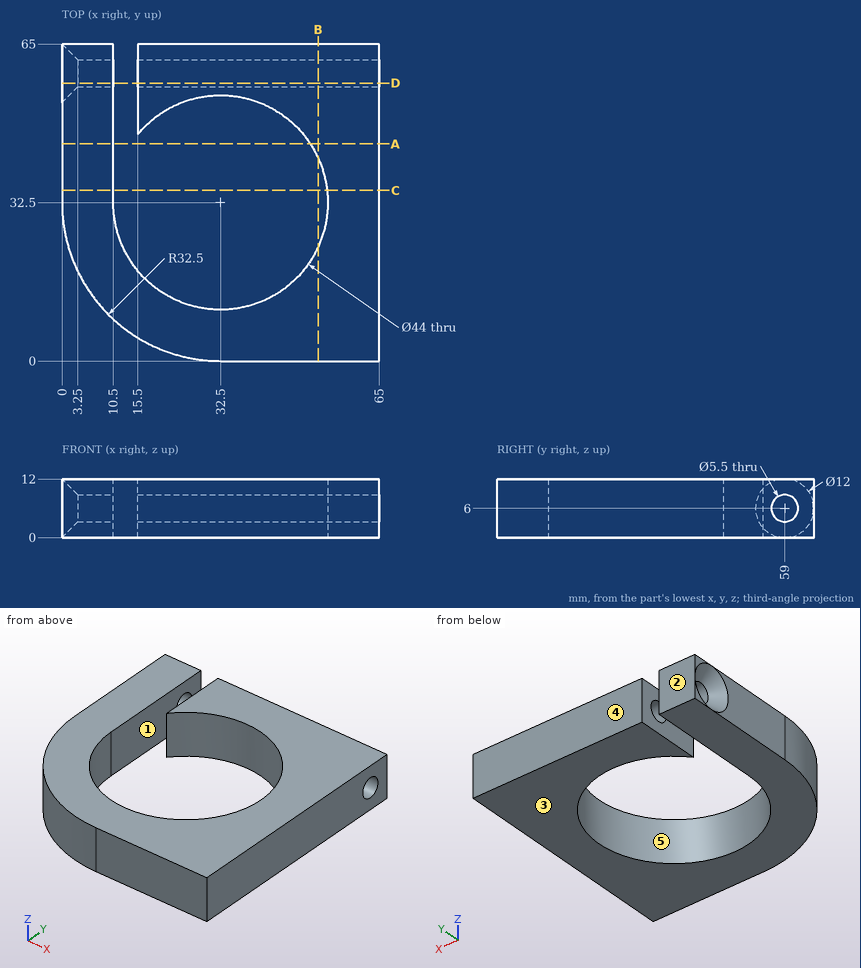
Here's the drawing with two shaded views (mm, measured from the low corner). I have some questions. A direction names the side the tool comes from. Coordinates: 2 decimals unless noted, no trailing zeros. Loops run counter-clockwise (first coordinate to the right, second up) from the corner with the lowest first, then second, coordinate; pieces in that order, holes last. Notation, with made-up numbers: M 76.5,46 L 101.5,46 A7 cw 101.5,57 Z; hole C 74,80.5 d7. An arc over 180 degrees is marked long. Answer as CSV lines item,"result". Start each with the question number.
1. Thinking about a two-plate mould opening in Y: for the marked faces 3, 4 and 5, which applies, +Y half, -Y half, draft (parallel to the pull), parting line (faces both ways), or undercut?
2. Suppose I cut it at A-A, the plane y = 44.5. List the corners of the cut face in (x, z) for me.
3. Suppose I cut it at B-B, the plane x = 52.5. List the corners of the cut face in (y, z) for me.
4. For pin 1 Ø1 at (y, z) = (30, 10) entering from -X, with a flat end and sliding along its axis, tell me the tip position at first contact or that it passes through.
5. Suppose I cut it at D-D, the plane y = 57. Count the separate pieces of the cut face and the enclosed holes in it, plus the area to 3 significant figures.
6. For the marked faces 1 and 2, which set-ups out of +Z, -Z, +X, -X, +Y, -Y let a thin tool reach every point of the face, with its end or its side?
7. Suppose I cut it at C-C, the plane y = 35. List the corners of the cut face in (x, z) for me.
8. If I drill on probe 1 along Y at (x, z) = (52, 7.75); probe 2 along Z at (x, y) = (8, 59); probe 3 along X at (y, z) = (51, 11.25), over which ranges is the centre line in solid material (lowest first)? Write a range as [from, to].
Output:
1,face 3,"draft"
1,face 4,"+Y half"
1,face 5,"undercut"
2,outline,"M 0,0 L 10.5,0 L 10.5,12 L 0,12 Z; M 50.94,0 L 65,0 L 65,12 L 50.94,12 Z"
3,outline,"M 0,0 L 23.33,0 L 23.33,12 L 0,12 Z; M 41.67,0 L 65,0 L 65,12 L 41.67,12 Z; hole C 59,6 d5.5"
4,pin 1,"stops at x = 0.06"
5,separate pieces,"4"
5,enclosed holes,"0"
5,area,"481 mm^2"
6,face 1,"+Z, -Z, +Y"
6,face 2,"+Z, -Z, +X, -X, +Y"
7,outline,"M 0,0 L 10.5,0 L 10.5,12 L 0,12 Z; M 54.36,0 L 65,0 L 65,12 L 54.36,12 Z"
8,probe 1,"y = [0, 22.31], [42.69, 56.88], [61.12, 65]"
8,probe 2,"z = [0, 3.25], [8.75, 12]"
8,probe 3,"x = [0, 10.5], [15.5, 20.59], [44.41, 65]"
